Geometry check sheet. Reference: the model listing, model coordinates, mm. A direction names the side the tool comes from. Coordinates: 2 decimals unless noted, no trailing zeros. Write each loop counter-clockwise with the first axis right and the second up, starting at its lowest first coordinate (ties: lowest second). Pieces come first, ordered by that corner, then holes.
from build123d import *
from build123d.topology import SkipClean

# Parameters (mm, degrees)
SKETCH1_R                = 7.874
BOSS_EXTRUDE1_DEPTH      = 50.8
CUT_EXTRUDE1_START       = -50.8
CUT_EXTRUDE1_OUTLINE_W   = 25.4
CUT_EXTRUDE1_OUTLINE_H   = 6.35
CUT_EXTRUDE1_OUTLINE_W_2 = 49.568192559
CUT_EXTRUDE1_OUTLINE_H_2 = 25.4
CUT_EXTRUDE1_OUTLINE_R   = 7.112
CUT_EXTRUDE1_DEPTH       = 50.8
SKETCH3_R                = 15.875
SKETCH3_R_2              = 6.921426928
BOSS_EXTRUDE2_DEPTH      = 6.35
BOSS_EXTRUDE3_START      = 6.35
SKETCH4_R                = 15.875
SKETCH4_R_2              = 7.112
BOSS_EXTRUDE3_DEPTH      = 6.35
SKETCH5_R                = 15.748
SKETCH5_R_2              = 7.874
BOSS_EXTRUDE4_DEPTH      = 6.35
BOSS_EXTRUDE5_START      = 6.35
SKETCH6_R                = 15.748
SKETCH6_R_2              = 7.874
BOSS_EXTRUDE5_DEPTH      = 6.35


# Read off the part's stored shape, not the designer's step: Cut-Extrude1
with BuildPart() as part:
    # Sketch1 → Boss-Extrude1 (new body)
    with BuildSketch(Plane(origin=(0, 0, 0), x_dir=(1, 0, 0), z_dir=(0, 1, 0))):
        with BuildLine():
            Line((-60.013493944, 26.069313577), (16.186506056, 26.069313577))
            Line((16.186506056, 26.069313577), (46.712972556, 15.559540077))
            ThreePointArc((46.712972556, 15.559540077), (57.334279676, 0.584874102), (46.55299975, -14.27503132))
            Line((46.55299975, -14.27503132), (16.186506056, -24.730686423))
            Line((16.186506056, -24.730686423), (-60.013493944, -24.730686423))
            Line((-60.013493944, -24.730686423), (-60.013493944, -12.030686423))
            Line((-60.013493944, -12.030686423), (3.486506056, -12.030686423))
            Line((3.486506056, -12.030686423), (3.486506056, 13.369313577))
            Line((3.486506056, 13.369313577), (-60.013493944, 13.369313577))
            Line((-60.013493944, 13.369313577), (-60.013493944, 26.069313577))
        make_face()
        with Locations(Location((41.586506056, 0.669313577, 0), (0, 0, 270))):
            Circle(SKETCH1_R, mode=Mode.SUBTRACT)
    extrude(amount=BOSS_EXTRUDE1_DEPTH)

    # Cut-Extrude1 outline → Cut-Extrude1 (cut)
    with BuildSketch(Plane.XY.offset(24.730686423).offset(CUT_EXTRUDE1_START)):
        with BuildLine():
            ThreePointArc((-60.013493944, 25.4), (-52.574006186, 43.360512242), (-34.613493944, 50.8))
            Line((-34.613493944, 50.8), (-60.013493944, 50.8))
            Line((-60.013493944, 50.8), (-60.013493944, 25.4))
        make_face()
        with BuildLine():
            ThreePointArc((-34.613493944, 0), (-52.574006186, 7.439487758), (-60.013493944, 25.4))
            Line((-60.013493944, 25.4), (-60.013493944, 0))
            Line((-60.013493944, 0), (-34.613493944, 0))
        make_face()
        with Locations((-9.213493944, 47.625)):
            Rectangle(CUT_EXTRUDE1_OUTLINE_W, CUT_EXTRUDE1_OUTLINE_H)
        with Locations((-9.213493944, 3.175)):
            Rectangle(CUT_EXTRUDE1_OUTLINE_W, CUT_EXTRUDE1_OUTLINE_H)
        with Locations((40.970602336, 25.4)):
            Rectangle(CUT_EXTRUDE1_OUTLINE_W_2, CUT_EXTRUDE1_OUTLINE_H_2)
        with Locations((-34.613493944, 25.4)):
            Circle(CUT_EXTRUDE1_OUTLINE_R)
    extrude(amount=CUT_EXTRUDE1_DEPTH, mode=Mode.SUBTRACT)

    # Sketch3 → Boss-Extrude2 (add)
    with BuildSketch(Plane.XY.offset(24.730686423)):
        with Locations((-34.613493944, 25.4)):
            Circle(SKETCH3_R)
        with Locations((-34.613493944, 25.4)):
            Circle(SKETCH3_R_2, mode=Mode.SUBTRACT)
    extrude(amount=BOSS_EXTRUDE2_DEPTH)

    # Sketch4 → Boss-Extrude3 (add)
    with SkipClean():  # the faces are left unmerged after this step: merging them gives an invalid solid
        with BuildSketch(Plane(origin=(0, 0, -26.069313577), x_dir=(-1, 0, 0), z_dir=(0, 0, -1)).offset(BOSS_EXTRUDE3_START)):
            with Locations(Location((34.613493944, 25.4, 0), (0, 0, 180))):
                Circle(SKETCH4_R)
            with Locations((34.613493944, 25.4)):
                Circle(SKETCH4_R_2, mode=Mode.SUBTRACT)
        extrude(amount=-BOSS_EXTRUDE3_DEPTH)

    # Sketch5 → Boss-Extrude4 (add)
    with SkipClean():  # the faces are left unmerged after this step: merging them gives an invalid solid
        with BuildSketch(Plane(origin=(0, 12.7, 0), x_dir=(1, 0, 0), z_dir=(0, 1, 0))):
            with Locations(Location((41.586506056, 0.669313577, 0), (0, 0, 71.002234849))):
                Circle(SKETCH5_R)
            with Locations(Location((41.586506056, 0.669313577, 0), (0, 0, 270))):
                Circle(SKETCH5_R_2, mode=Mode.SUBTRACT)
        extrude(amount=BOSS_EXTRUDE4_DEPTH)

    # Sketch6 → Boss-Extrude5 (add)
    with SkipClean():  # the faces are left unmerged after this step: merging them gives an invalid solid
        with BuildSketch(Plane.XZ.offset(-38.1).offset(BOSS_EXTRUDE5_START)):
            with Locations(Location((41.586506056, -0.669313577, 0), (0, 0, 288.997765151))):
                Circle(SKETCH6_R)
            with Locations(Location((41.586506056, -0.669313577, 0), (0, 0, 90))):
                Circle(SKETCH6_R_2, mode=Mode.SUBTRACT)
        extrude(amount=-BOSS_EXTRUDE5_DEPTH)
    add(part.part.scale(1), mode=Mode.REPLACE)  # the faces are merged on a copy


solid = part.part
1. Sectioned sample at B-B, the plane x = -38.5. Record the boundary of the cut face in (y, z), and give its area (3 significant figures).
Computed values:
outline: (0.3, -26.07) - (10.01, -26.07) - (10.01, -32.42) - (19.44, -32.42) - (19.44, -13.37) - (0.3, -13.37) - close; (0.3, 12.03) - (19.44, 12.03) - (19.44, 24.73) - (19.67, 24.73) - (19.67, 31.08) - (10.01, 31.08) - (10.01, 24.73) - (0.3, 24.73) - close; (31.13, 24.73) - (31.36, 24.73) - (31.36, 12.03) - (50.5, 12.03) - (50.5, 24.73) - (40.79, 24.73) - (40.79, 31.08) - (31.13, 31.08) - close; (31.36, -32.42) - (40.79, -32.42) - (40.79, -26.07) - (50.5, -26.07) - (50.5, -13.37) - (31.36, -13.37) - close
area: 1,220 mm2
2. Sectioned sample at A-A, the plane y = 46.5. Record the boundary of the cut face in (x, z).
Computed values:
outline: (-48.75, -26.07) - (-21.91, -26.07) - (-21.91, -13.37) - (-48.75, -13.37) - close; (-48.75, 12.03) - (-21.91, 12.03) - (-21.91, 24.73) - (-48.75, 24.73) - close; (3.49, -26.07) - (16.19, -26.07) - (46.71, -15.56) arc R15.75 ccw to (46.55, 14.28) - (16.19, 24.73) - (3.49, 24.73) - close; hole circle Ø15.75 at (41.59, -0.67)
3. Sectioned sample at C-C, the plane z = -19. Record the boundary of the cut face in (x, y), and give its area (3 significant figures).
Computed values:
outline: (-34.61, 0) - (-21.91, 0) - (-21.91, 6.35) - (3.49, 6.35) - (3.49, 0) - (36.72, 0) - (36.72, 12.7) - (16.19, 12.7) - (16.19, 38.1) - (36.72, 38.1) - (36.72, 50.8) - (3.49, 50.8) - (3.49, 44.45) - (-21.91, 44.45) - (-21.91, 50.8) - (-34.61, 50.8) arc R25.4 ccw to start; hole circle Ø14.22 at (-34.61, 25.4)
area: 3,630 mm2
4. Access from +Z, -Z, +X, -X, +Y, -Y to the whole of each face (thin tool, end or side, straight path). Record for faces 4 (the flat face through (-9, 44.45, -20)), 5 (the cylindrical face through (-26.1, 12, -29.3)), 6 (the flat face through (16.187, 25, -1)).
Computed values:
face 4: +Z, -Z, +Y
face 5: -Z
face 6: +Z, -Z
5. Sectioned sample at D-D, the plane y = 20.5. Record the boundary of the cut face in (x, z), and give its area (3 significant figures).
Computed values:
outline: (-59.54, -26.07) - (-49.71, -26.07) - (-49.71, -32.42) - (-39.77, -32.42) - (-39.77, -13.37) - (-59.54, -13.37) - close; (-59.54, 12.03) - (-39.77, 12.03) - (-39.77, 24.73) - (-39.5, 24.73) - (-39.5, 31.08) - (-49.71, 31.08) - (-49.71, 24.73) - (-59.54, 24.73) - close; (-29.73, 24.73) - (-29.46, 24.73) - (-29.46, 12.03) - (3.49, 12.03) - (3.49, -13.37) - (-29.46, -13.37) - (-29.46, -32.42) - (-19.51, -32.42) - (-19.51, -26.07) - (16.19, -26.07) - (16.19, 24.73) - (-19.51, 24.73) - (-19.51, 31.08) - (-29.73, 31.08) - close
area: 2,240 mm2
6. Gauge pin test, flat ends, axial feed: pin 1 Ø4 at (x, z) = (-6.5, 20) entering from -Y; pin 2 Ø2 at (y, z) = (5.5, -20) entering from -X; pin 3 Ø12 at (x, y) = (8, 39) entering from -Z; pin 4 Ø4 at (x, z) = (-22.5, 9.5) entering from +Y. Record the tip position at first contact, or that the pin passes through.
Computed values:
pin 1: stops at y = 6.35
pin 2: stops at x = -51.58
pin 3: stops at z = -26.07
pin 4: passes through
7. Thickness scan on line 1 along Z through (x, y) = (-9, 15); line 2 along X through (y, z) = (25, -30); line 3 along Y through (x, z) = (29, -15). Record the ranges inside material, lowest first.
Computed values:
line 1: z = -26.07 to -13.37, 12.03 to 24.73
line 2: x = -50.48 to -41.71, -27.51 to -18.74
line 3: y = 0 to 12.7, 38.1 to 50.8
8. Draft check along Z on faces 1 (the flat face through (-31, 19, 31.081)), 2 (the flat face through (3.487, 25, -1)), 3 (the flat face through (-28, 50.8, 18)). Enter one of: released by +Z, released by -Z, zero draft, split by the parting line, or undercut.
Computed values:
face 1: released by +Z
face 2: undercut
face 3: zero draft
